```python
from build123d import *

# Parameters (mm, degrees)
F0_R     = 6.35
F1_DEPTH = 76.2
F3_DEPTH = 25.4
F4_R     = 1.5875
F5_DEPTH = 25.4


with BuildPart() as f1:
    # F0 (on Front) → F1 (new body)
    with BuildSketch(Plane.XZ):
        Circle(F0_R)
    extrude(amount=F1_DEPTH)

    # F2 (on face) → F3 (cut)
    with BuildSketch(Plane.XZ.offset(76.2)):
        with BuildLine():
            ThreePointArc((3.81, -5.08), (6.35, 0), (3.81, 5.08))
            Line((3.81, 5.08), (3.81, -5.08))
        make_face()
        with BuildLine():
            Line((-3.81, -5.08), (-3.81, 5.08))
            ThreePointArc((-3.81, 5.08), (-6.35, 0), (-3.81, -5.08))
        make_face()
    extrude(amount=-F3_DEPTH, mode=Mode.SUBTRACT)

    # F4 (on face) → F5 (cut)
    with BuildSketch(Plane.YZ.offset(3.81)):
        with Locations((-69.85, 0)):
            Circle(F4_R)
    extrude(amount=-F5_DEPTH, mode=Mode.SUBTRACT)


solid = f1.part
```
Could you check a few things on this model? Use its own coordinates, in mm. A direction names the side the tool comes from. Round coordinates to 2 decimals unless told otherwise and drop trailing zeros. Order: outer loops, then holes, each group sorted by start corner. A loop starts at its lowest first (then second) coordinate and runs counter-clockwise, first axis right, second up. Notation, with made-up numbers: (-32, -34) -> (-24, -34) arc R20 ccw to (-24, -5) -> close; hole circle Ø1 at (-6.5, -23). An arc over 180 degrees is marked (long way). One line per question, with ' | ' between items.
Q1. If I drill on line 1 (Z direction, x = 0, y = -69.85); line 2 (Y direction, x = -5.75, z = -2); line 3 (Y direction, x = 3.25, z = 1), over which ranges is the centre line in solid material (lowest first)? Write a range as from..to.
Computed values:
line 1: -6.35..-1.59, 1.59..6.35 | line 2: -50.8..0 | line 3: -76.2..-71.08, -68.62..0
Q2. If we section it at D-D on z = 4.25: Write out the boundary of the cut face in (x, y).
Computed values:
outline: (-4.72, -50.8) -> (-3.81, -50.8) -> (-3.81, -76.2) -> (3.81, -76.2) -> (3.81, -50.8) -> (4.72, -50.8) -> (4.72, 0) -> (-4.72, 0) -> close
Q3. Which directions (+Z, -Z, +X, -X, +Y, -Y) give clear straight access to the entire face, cutting with the end or side of a thin tool? Please do faces 1 (the face through (-5, -50.8, 0)), 2 (the face through (3.81, -64, 0)), 3 (the face through (0, 0, 0)).
Computed values:
face 1: +Z, -Z, -X, -Y | face 2: +Z, -Z, +X, -Y | face 3: +Z, -Z, +X, -X, +Y
Q4. If we section it at A-A on y = -69.85: Write out the boundary of the cut face in (x, z).
Computed values:
outline: (-3.81, -5.08) arc R6.35 ccw to (3.81, -5.08) -> (3.81, -1.59) -> (-3.81, -1.59) -> close; (-3.81, 1.59) -> (3.81, 1.59) -> (3.81, 5.08) arc R6.35 ccw to (-3.81, 5.08) -> close
Q5. If we section it at B-B on z = 0: Write out the boundary of the cut face in (x, y), plus the area to 3 significant figures.
Computed values:
outline: (-6.35, -50.8) -> (-3.81, -50.8) -> (-3.81, -68.26) -> (3.81, -68.26) -> (3.81, -50.8) -> (6.35, -50.8) -> (6.35, 0) -> (-6.35, 0) -> close; (-3.81, -76.2) -> (3.81, -76.2) -> (3.81, -71.44) -> (-3.81, -71.44) -> close | area: 815 mm²
Q6. We'd pull the mould along Z, two halves only. Please class faces 4 (the face through (5.866, -29.1, -2.432)), 5 (the face through (0, -76.2, 0)), 6 (the face through (0.053, -68.384, -0.608)): released by +Z, released by -Z, zero draft, split by the parting line, or undercut.
Computed values:
face 4: split by the parting line | face 5: zero draft | face 6: undercut
Q7. I'm going to push flat-ended pins straight in: pin 1 (3 mm diameter, centred on x = -3.5, y = -56, fed in from -Z); pin 2 (2 mm diameter, centred on x = -3.5, z = 3, fed in from +Y); pin 3 (5 mm diameter, centred on y = -69.85, z = 0, fed in from +X); pin 4 (0.8 mm diameter, centred on x = -5.5, z = 0.5, fed in from -Y). Where does each tip first touch, or does it pass through?
Computed values:
pin 1: z = -6.03 | pin 2: y = 0 | pin 3: x = 3.81 | pin 4: y = -50.8
